from build123d import *

# Parameters (mm, degrees)
CROQUIS1_W              = 135
CROQUIS1_H              = 50
CROQUIS1_R              = 1.65
CROQUIS1_R_2            = 1.6
SALIENTE_EXTRUIR1_DEPTH = 4
CROQUIS2_W              = 135
CROQUIS2_H              = 50
SALIENTE_EXTRUIR2_DEPTH = 2
CROQUIS3_W              = 135
CROQUIS3_H              = 50
CROQUIS3_R              = 0.85
SALIENTE_EXTRUIR3_DEPTH = 6


with BuildPart() as part:
    # Croquis1 → Saliente-Extruir1 (new body)
    with BuildSketch(Plane.XY):
        with Locations((0.24843477, -0.062108693)):
            Rectangle(CROQUIS1_W, CROQUIS1_H)
        with Locations((-57.493419725, 15.937891307)):
            Circle(CROQUIS1_R, mode=Mode.SUBTRACT)
        with Locations((-25.493419725, 15.937891307)):
            Circle(CROQUIS1_R, mode=Mode.SUBTRACT)
        with Locations((-25.493419725, -16.062108693)):
            Circle(CROQUIS1_R, mode=Mode.SUBTRACT)
        with Locations((-57.493419725, -16.062108693)):
            Circle(CROQUIS1_R, mode=Mode.SUBTRACT)
        with Locations((28.686131392, -0.062108693)):
            Circle(CROQUIS1_R_2, mode=Mode.SUBTRACT)
        with Locations((-11.313868608, -0.062108693)):
            Circle(CROQUIS1_R_2, mode=Mode.SUBTRACT)
        Polygon((59.170162083, 12.86736071), (39.870162083, 12.86736071), (39.870162083, -12.93263929), (39.920162083, -12.93263929), (39.920162083, -12.991578095), (59.120162083, -12.991578095), (59.120162083, -12.93263929), (59.170162083, -12.93263929), align=None, mode=Mode.SUBTRACT)
        with BuildLine():
            Line((16.192628508, 8.387891307), (1.179634277, 8.387891307))
            Line((1.179634277, 8.387891307), (-3.863868608, 3.344388423))
            Line((-3.863868608, 3.344388423), (-3.863868608, -6.112108693))
            ThreePointArc((-3.863868608, -6.112108693), (-3.160924883, -7.809164967), (-1.463868608, -8.512108693))
            Line((-1.463868608, -8.512108693), (18.836131392, -8.512108693))
            ThreePointArc((18.836131392, -8.512108693), (20.533187667, -7.809164967), (21.236131392, -6.112108693))
            Line((21.236131392, -6.112108693), (21.236131392, 3.344388423))
            Line((21.236131392, 3.344388423), (16.192628508, 8.387891307))
        make_face(mode=Mode.SUBTRACT)
        with BuildLine():
            Line((-38.358377873, -0.368723419), (-35.225212961, -3.501888332))
            ThreePointArc((-35.225212961, -3.501888332), (-34.343419725, -0.062108693), (-35.225212961, 3.377670947))
            Line((-35.225212961, 3.377670947), (-38.358377873, 0.244506034))
            ThreePointArc((-38.358377873, 0.244506034), (-38.343419725, -0.062108693), (-38.358377873, -0.368723419))
        make_face(mode=Mode.SUBTRACT)
        with BuildLine():
            Line((-44.628461576, -0.368723419), (-47.761626488, -3.501888332))
            ThreePointArc((-47.761626488, -3.501888332), (-48.643419725, -0.062108693), (-47.761626488, 3.377670947))
            Line((-47.761626488, 3.377670947), (-44.628461576, 0.244506034))
            ThreePointArc((-44.628461576, 0.244506034), (-44.643419725, -0.062108693), (-44.628461576, -0.368723419))
        make_face(mode=Mode.SUBTRACT)
        with BuildLine():
            Line((-29.440590182, 14.819147975), (-32.288723267, 11.971014889))
            ThreePointArc((-32.288723267, 11.971014889), (-41.493419725, 15.087891307), (-50.698116182, 11.971014889))
            Line((-50.698116182, 11.971014889), (-53.546249267, 14.819147975))
            ThreePointArc((-53.546249267, 14.819147975), (-41.493419725, 19.087891307), (-29.440590182, 14.819147975))
        make_face(mode=Mode.SUBTRACT)
        with BuildLine():
            Line((-26.612163057, 11.99072085), (-29.460296143, 9.142587764))
            ThreePointArc((-29.460296143, 9.142587764), (-26.343419725, -0.062108693), (-29.460296143, -9.26680515))
            Line((-29.460296143, -9.26680515), (-26.612163057, -12.114938235))
            ThreePointArc((-26.612163057, -12.114938235), (-22.343419725, -0.062108693), (-26.612163057, 11.99072085))
        make_face(mode=Mode.SUBTRACT)
        with BuildLine():
            Line((-56.374676392, 11.99072085), (-53.526543306, 9.142587764))
            ThreePointArc((-53.526543306, 9.142587764), (-56.643419725, -0.062108693), (-53.526543306, -9.26680515))
            Line((-53.526543306, -9.26680515), (-56.374676392, -12.114938235))
            ThreePointArc((-56.374676392, -12.114938235), (-60.643419725, -0.062108693), (-56.374676392, 11.99072085))
        make_face(mode=Mode.SUBTRACT)
        with BuildLine():
            Line((-41.800034451, -3.197150544), (-44.933199364, -6.330315456))
            ThreePointArc((-44.933199364, -6.330315456), (-41.493419725, -7.212108693), (-38.053640085, -6.330315456))
            Line((-38.053640085, -6.330315456), (-41.186804998, -3.197150544))
            ThreePointArc((-41.186804998, -3.197150544), (-41.493419725, -3.212108693), (-41.800034451, -3.197150544))
        make_face(mode=Mode.SUBTRACT)
        with BuildLine():
            Line((-30.888925971, 7.713957937), (-33.765629521, 4.837254386))
            ThreePointArc((-33.765629521, 4.837254386), (-32.343419725, -0.062108693), (-33.765629521, -4.961471771))
            Line((-33.765629521, -4.961471771), (-30.888925971, -7.838175322))
            ThreePointArc((-30.888925971, -7.838175322), (-28.343419725, -0.062108693), (-30.888925971, 7.713957937))
        make_face(mode=Mode.SUBTRACT)
        with BuildLine():
            Line((-33.717353095, 10.542385061), (-36.594056646, 7.665681511))
            ThreePointArc((-36.594056646, 7.665681511), (-41.493419725, 9.087891307), (-46.392782803, 7.665681511))
            Line((-46.392782803, 7.665681511), (-49.269486354, 10.542385061))
            ThreePointArc((-49.269486354, 10.542385061), (-41.493419725, 13.087891307), (-33.717353095, 10.542385061))
        make_face(mode=Mode.SUBTRACT)
        with BuildLine():
            Line((-52.097913478, 7.713957937), (-49.221209928, 4.837254386))
            ThreePointArc((-49.221209928, 4.837254386), (-50.643419725, -0.062108693), (-49.221209928, -4.961471771))
            Line((-49.221209928, -4.961471771), (-52.097913478, -7.838175322))
            ThreePointArc((-52.097913478, -7.838175322), (-54.643419725, -0.062108693), (-52.097913478, 7.713957937))
        make_face(mode=Mode.SUBTRACT)
        with BuildLine():
            Line((-50.698116182, -12.095232274), (-53.546249267, -14.94336536))
            ThreePointArc((-53.546249267, -14.94336536), (-41.493419725, -19.212108693), (-29.440590182, -14.94336536))
            Line((-29.440590182, -14.94336536), (-32.288723267, -12.095232274))
            ThreePointArc((-32.288723267, -12.095232274), (-41.493419725, -15.212108693), (-50.698116182, -12.095232274))
        make_face(mode=Mode.SUBTRACT)
        with BuildLine():
            Line((-36.594056646, -7.789898896), (-33.717353095, -10.666602447))
            ThreePointArc((-33.717353095, -10.666602447), (-41.493419725, -13.212108693), (-49.269486354, -10.666602447))
            Line((-49.269486354, -10.666602447), (-46.392782803, -7.789898896))
            ThreePointArc((-46.392782803, -7.789898896), (-41.493419725, -9.212108693), (-36.594056646, -7.789898896))
        make_face(mode=Mode.SUBTRACT)
        with BuildLine():
            Line((-44.933199364, 6.206098071), (-41.800034451, 3.072933159))
            ThreePointArc((-41.800034451, 3.072933159), (-41.493419725, 3.087891307), (-41.186804998, 3.072933159))
            Line((-41.186804998, 3.072933159), (-38.053640085, 6.206098071))
            ThreePointArc((-38.053640085, 6.206098071), (-41.493419725, 7.087891307), (-44.933199364, 6.206098071))
        make_face(mode=Mode.SUBTRACT)
    extrude(amount=SALIENTE_EXTRUIR1_DEPTH)

    # Croquis2 → Saliente-Extruir2 (add)
    with BuildSketch(Plane.XY.offset(4)):
        with BuildLine():
            Line((70.74843477, -25.062108693), (70.74843477, 24.937891307))
            ThreePointArc((70.74843477, 24.937891307), (69.869755114, 27.059211651), (67.74843477, 27.937891307))
            Line((67.74843477, 27.937891307), (-67.25156523, 27.937891307))
            ThreePointArc((-67.25156523, 27.937891307), (-69.372885573, 27.059211651), (-70.25156523, 24.937891307))
            Line((-70.25156523, 24.937891307), (-70.25156523, -25.062108693))
            ThreePointArc((-70.25156523, -25.062108693), (-69.372885573, -27.183429036), (-67.25156523, -28.062108693))
            Line((-67.25156523, -28.062108693), (67.74843477, -28.062108693))
            ThreePointArc((67.74843477, -28.062108693), (69.869755114, -27.183429036), (70.74843477, -25.062108693))
        make_face()
        with Locations((0.24843477, -0.062108693)):
            Rectangle(CROQUIS2_W, CROQUIS2_H, mode=Mode.SUBTRACT)
    extrude(amount=-SALIENTE_EXTRUIR2_DEPTH)

    # Croquis3 → Saliente-Extruir3 (add)
    with BuildSketch(Plane(origin=(0, 0, 0), x_dir=(-1, 0, 0), z_dir=(0, 0, -1))):
        with Locations((-0.24843477, -0.062108693)):
            Rectangle(CROQUIS3_W, CROQUIS3_H)
        with Locations((-64.99843477, 22.187891307)):
            Circle(CROQUIS3_R, mode=Mode.SUBTRACT)
        with Locations((64.50156523, 22.187891307)):
            Circle(CROQUIS3_R, mode=Mode.SUBTRACT)
        with Locations((-64.99843477, -22.312108693)):
            Circle(CROQUIS3_R, mode=Mode.SUBTRACT)
        with Locations((64.50156523, -22.312108693)):
            Circle(CROQUIS3_R, mode=Mode.SUBTRACT)
        Polygon((-64.74843477, 16.937891307), (-64.74843477, -17.062108693), (-59.74843477, -22.062108693), (59.25156523, -22.062108693), (64.25156523, -17.062108693), (64.25156523, 16.937891307), (59.25156523, 21.937891307), (-59.74843477, 21.937891307), align=None, mode=Mode.SUBTRACT)
    extrude(amount=SALIENTE_EXTRUIR3_DEPTH)


solid = part.part
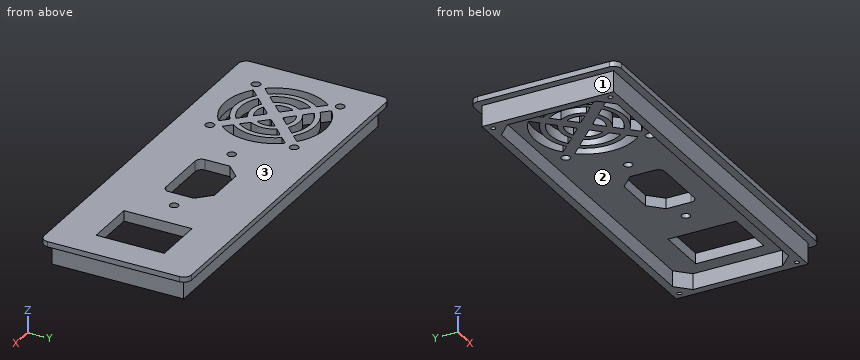
The model under review builds one solid part; all positions refer to its coordinate system, in mm. Face numbers are marked on the shaded views. Round coordinates to 2 decimals unless told otherwise and drop trailing zeros. Write each loop counter-clockwise with the first axis right and the second up, starting at its lowest first coordinate (ties: lowest second). Pieces come first, ordered by that corner, then holes. Notation, with made-up numbers: M 23.25,89 L 80.25,89 A17 ccw 80.25,109 Z; hole C 36,-21 d10. An arc over 180 degrees is marked long. Use a Markdown table: item, result. Add a question column.
Q1. We need section B-B, the plane z = -3. State the section outline as (x, y) points, plus the area to 3 significant figures.
Q2. To check wall thickness, follow line 1 (Y direction, x = 55.5, z = -2.75); line 2 (X direction, y = 13.5, z = -2); line 3 (X direction, y = -22, z = -2). State the ranges of each line that lie inside material, in increasing order.
Q3. The part is to be moulded in two halves that separate along X. For the marked faces 1, 2 and 3, say which applies: pulls with the +X half, pulls with the -X half, needs draft (parallel to the pull), parting line crosses it, or undercut.
Q4. Insertion check: pin 1 (5 mm diameter, centred on x = -4.5, z = -4, fed in from +Y); pin 2 (1 mm diameter, centred on x = -64.5, y = 22.19, fed in from -Z); pin 3 (4 mm diameter, centred on x = 18, z = -2, fed in from -Y); pin 4 (2.5 mm diameter, centred on x = -57.49, y = -16.06, fed in from +Z). Each pin has a flat end and moves straight along its axis. Give the tip position at first contact, or say it passes through.
Q5. We need section A-A, the plane x = -15.5. State the section outline as (y, z) points, plus the area to 3 significant figures.
Findings below:
| question | item | result |
|---|---|---|
| 1 | outline | M -67.25,-25.06 L 67.75,-25.06 L 67.75,24.94 L -67.25,24.94 Z; hole C -64.5,-22.31 d1.7; hole C -64.5,22.19 d1.7; hole M -64.25,-17.06 L -59.25,-22.06 L 59.75,-22.06 L 64.75,-17.06 L 64.75,16.94 L 59.75,21.94 L -59.25,21.94 L -64.25,16.94 Z; hole C 65,-22.31 d1.7; hole C 65,22.19 d1.7 |
| 1 | area | 1,110 mm² |
| 2 | line 1 | y = -25.06 to -22.06, 21.94 to 24.94 |
| 2 | line 2 | x = -67.25 to -64.25, 64.75 to 67.75 |
| 2 | line 3 | x = -67.25 to -65.29, -63.71 to -59.31, 59.81 to 64.21, 65.79 to 67.75 |
| 3 | face 1 | pulls with the -X half |
| 3 | face 2 | undercut |
| 3 | face 3 | needs draft |
| 4 | pin 1 | stops at y = 24.94 |
| 4 | pin 2 | stops at z = 0 |
| 4 | pin 3 | stops at y = -25.06 |
| 4 | pin 4 | passes through |
| 5 | outline | M -28.06,2 L -25.06,2 L -25.06,-6 L -22.06,-6 L -22.06,0 L 21.94,0 L 21.94,-6 L 24.94,-6 L 24.94,2 L 27.94,2 L 27.94,4 L -28.06,4 Z |
| 5 | area | 248 mm² |
